Geometry: see drawing. Coordinates: mm, zero at the bounding-box minimum. Give positions to 0.01 mm unless a question says otherwise; leave off trailing zeros. Order: outer loops, then holes, each group sorted by start corner. A loop starts at its lowest first (then second) coordinate and runs counter-clockwise, first axis right, second up. Notation, with made-up numbers: M -12.75,-30 L 26.25,-30 A23 ccw 26.25,2 Z; hole C 10.25,25.25 d10. An arc over 180 degrees is marked long. Return JSON: item names as keys, results as strings.
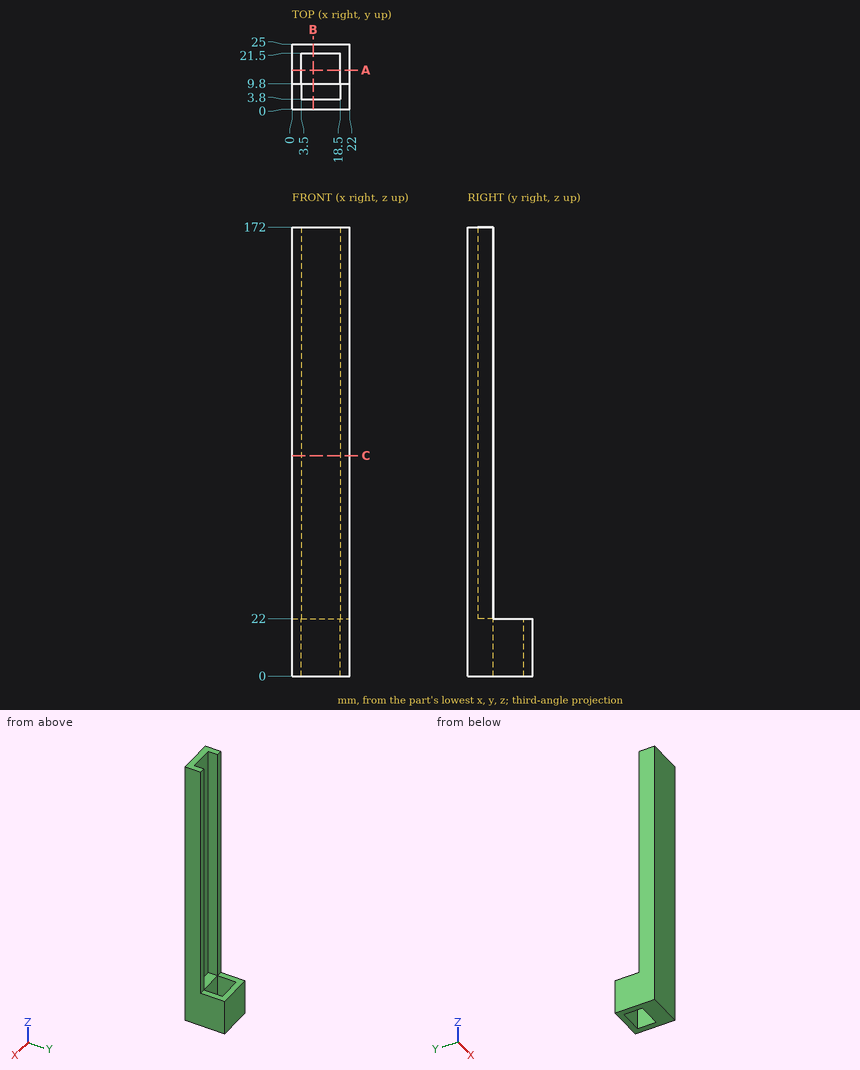
1. Section query A-A (y = 15). Return loops of the section in (x, z), then the cut area to 3 significant figures.
Evaluation:
{"outline": "M 0,0 L 3.5,0 L 3.5,22 L 0,22 Z; M 18.5,0 L 22,0 L 22,22 L 18.5,22 Z", "area": "154 mm^2"}
2. Section query C-C (z = 84.5). Return loops of the section in (x, y).
Evaluation:
{"outline": "M 0,0 L 22,0 L 22,9.8 L 18.5,9.8 L 18.5,3.8 L 3.5,3.8 L 3.5,9.8 L 0,9.8 Z"}
3. Section query B-B (x = 8). Return loops of the section in (y, z).
Evaluation:
{"outline": "M 0,0 L 9.8,0 L 9.8,22 L 3.8,22 L 3.8,172 L 0,172 Z; M 21.5,0 L 25,0 L 25,22 L 21.5,22 Z"}
4. Ray query, probe 1 along Y at (x, z) = (12.75, 13.5); probe 2 along X at (y, z) = (5.5, 60); probe 3 along Y at (x, z) = (13.25, 165). Return the intervals inside material, ascending.
Evaluation:
{"probe 1": "y = 0 to 9.8, 21.5 to 25", "probe 2": "x = 0 to 3.5, 18.5 to 22", "probe 3": "y = 0 to 3.8"}
5. First-contact query: pin 1 (1.1 mm diameter, centred on x = 1, z = 107, fed in from +Y); pin 2 (5 mm diameter, centred on x = 10.5, z = 154.5, fed in from +Y); pin 3 (10 mm diameter, centred on x = 16, y = 21.5, fed in from +Z). Flat tips, straight axial feed; report the tip coordinate or a pass-through.
Evaluation:
{"pin 1": "stops at y = 9.8", "pin 2": "stops at y = 3.8", "pin 3": "stops at z = 22"}
